Part model, mm, in its own coordinate system. Face numbers are marked on the shaded views. Round coordinates to 2 decimals unless told otherwise and drop trailing zeros. Write each loop counter-clockwise with the first axis right and the second up, starting at its lowest first coordinate (ties: lowest second). Pieces come first, ordered by that corner, then holes. Notation, with made-up numbers: M -18,22.5 L 23,22.5 A22 ccw 23,39.5 Z; hole C 48.5,41 d10. An arc over 180 degrees is marked long. Answer as a JSON object with one key per item and string values. Group by question number.
1. Band-saw the part on B-B, the plane x = 0. Write the cut outline in (y, z), plus the area to 3 significant figures.
2. Drill centre lines: line 1 (Y direction, x = 12.5, z = 5); line 2 (Y direction, x = 0.5, z = 1.05); line 3 (Y direction, x = -27.5, z = 4.8). Where is each one in solid material? Low to high. Write a range as from..to.
3. Two-plate mould, pull along X, no slides. Class the marked faces 1, 2 and 3: +X half, -X half, draft (parallel to the pull), parting line (faces both ways), or undercut.
4. Band-saw the part on D-D, the plane z = 2.15. Write the cut outline in (x, y), plus the area to 3 significant figures.
5. Drop flat-ended pins along their axis: pin 1 (1 mm diameter, centred on x = -10.5, y = 20.5, fed in from -Z); pin 2 (1.5 mm diameter, centred on y = -14.5, z = 3.5, fed in from +X); pin 3 (3 mm diameter, centred on x = -11, z = 1, fed in from -Y); pin 4 (3.5 mm diameter, centred on x = -21.58, y = 17.21, fed in from -Z). Give the stop position or say it passes through.
6. Band-saw the part on C-C, the plane x = -18. Write the cut outline in (y, z), plus the area to 3 significant figures.
7. Band-saw the part on A-A, the plane y = 0. Write the cut outline in (x, z).
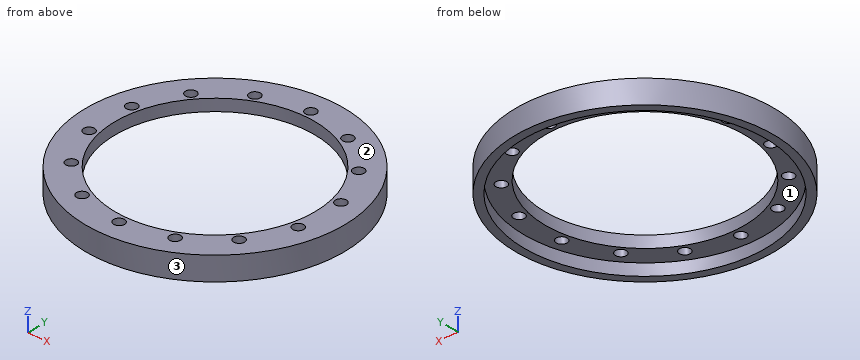
from build123d import *

# Parameters (mm, degrees)
SKETCH_R           = 33
PAD_DEPTH          = 6
SKETCH001_R        = 25.5
POCKET_DEPTH       = 6.001
SKETCH002_R        = 1.4
POCKET001_DEPTH    = 193.062487
POLARPATTERN_COUNT = 14
SKETCH004_R        = 30.9
POCKET002_DEPTH    = 3


with BuildPart() as part:
    # Sketch → Pad (new body)
    with BuildSketch(Plane.XY):
        Circle(SKETCH_R)
    extrude(amount=PAD_DEPTH)

    # Sketch001 → Pocket (cut, through all)
    with BuildSketch(Plane.XY.offset(6)):
        Circle(SKETCH001_R)
    extrude(amount=-POCKET_DEPTH, mode=Mode.SUBTRACT)

    # Sketch002 → Pocket001 (cut, through all)
    with BuildSketch(Plane.XY.offset(6)):
        with Locations((0, 27.6)):
            Circle(SKETCH002_R)
    pocket001 = extrude(amount=-POCKET001_DEPTH, mode=Mode.SUBTRACT)

    # PolarPattern: Pocket001 ×14 about axis
    polarpattern_axis = Axis((0, 0, 6), (0, 0, 1))
    for i in range(1, POLARPATTERN_COUNT):
        add(pocket001.rotate(polarpattern_axis, i * 360 / POLARPATTERN_COUNT), mode=Mode.SUBTRACT)

    # Sketch004 → Pocket002 (cut)
    with BuildSketch(Plane(origin=(0, 0, 0), x_dir=(1, 0, 0), z_dir=(0, 0, -1))):
        Circle(SKETCH004_R)
    extrude(amount=-POCKET002_DEPTH, mode=Mode.SUBTRACT)


solid = part.part
Worked answers:
{
 "1": {"outline": "M -33,0 L -30.9,0 L -30.9,3 L -29,3 L -29,6 L -33,6 Z; M -26.2,3 L -25.5,3 L -25.5,6 L -26.2,6 Z; M 25.5,3 L 26.2,3 L 26.2,6 L 25.5,6 Z; M 29,3 L 30.9,3 L 30.9,0 L 33,0 L 33,6 L 29,6 Z", "area": "40.8 mm^2"},
 "2": {"line 1": "y = -30.54..-26.16, -23.57..-22.23, 22.23..23.57, 26.16..30.54", "line 2": "y = -33..-30.9, 30.9..33", "line 3": "y = -18.24..-7.41, -4.87..4.87, 7.41..18.24"},
 "3": {"face 1": "undercut", "face 2": "draft", "face 3": "parting line"},
 "4": {"outline": "C 0,0 d66; hole C 0,0 d61.8", "area": "422 mm^2"},
 "5": {"pin 1": "passes through", "pin 2": "stops at x = 30", "pin 3": "stops at y = -31.6", "pin 4": "stops at z = 3"},
 "6": {"outline": "M -27.66,0 L -25.12,0 L -25.12,3 L -18.06,3 L -18.06,6 L -27.66,6 Z; M 18.06,3 L 25.12,3 L 25.12,0 L 27.66,0 L 27.66,6 L 18.06,6 Z", "area": "72.8 mm^2"},
 "7": {"outline": "M -33,0 L -30.9,0 L -30.9,3 L -25.5,3 L -25.5,6 L -33,6 Z; M 25.5,3 L 30.9,3 L 30.9,0 L 33,0 L 33,6 L 25.5,6 Z"}
}
